Build history of the part. All positions in model axes, mm. Face numbers are marked on the shaded views. A direction names the side the tool comes from. Coordinates: 2 decimals unless noted, no trailing zeros. Order: outer loops, then holes, each group sorted by start corner. A loop starts at its lowest first (then second) coordinate and runs counter-clockwise, first axis right, second up. Notation, with made-up numbers: (-4, 36.5) - (38, 36.5) arc R17 ccw to (38, 41.5) - close; hole circle Ø4 at (17.5, 15.5). An arc over 180 degrees is marked (long way). Return JSON: item names as keys, results as strings.
from build123d import *

# Parameters (mm, degrees)
SKETCH1_W           = 457.2
SKETCH1_H           = 1244.6
BOSS_EXTRUDE1_DEPTH = 63.5
SKETCH4_W           = 457.2
SKETCH4_H           = 63.5
BOSS_EXTRUDE2_DEPTH = 266.7
CUT_EXTRUDE7_DEPTH  = 100.076
SKETCH12_W          = 63.5
SKETCH12_H          = 1244.6
CUT_EXTRUDE8_DEPTH  = 253.746


with BuildPart() as part:
    # Sketch1 → Boss-Extrude1 (new body)
    with BuildSketch(Plane(origin=(0, 0, 0), x_dir=(1, 0, 0), z_dir=(0, 1, 0))):
        with Locations((228.6, 622.3)):
            Rectangle(SKETCH1_W, SKETCH1_H)
    extrude(amount=BOSS_EXTRUDE1_DEPTH)

    # Sketch4 → Boss-Extrude2 (add)
    with BuildSketch(Plane(origin=(0, 63.5, 0), x_dir=(1, 0, 0), z_dir=(0, 1, 0))):
        with Locations((228.6, 1212.85)):
            Rectangle(SKETCH4_W, SKETCH4_H)
    boss_extrude2 = extrude(amount=BOSS_EXTRUDE2_DEPTH)

    # Mirror7: Boss-Extrude2 across plane
    add(boss_extrude2.mirror(Plane(origin=(0, 0, -622.3), x_dir=(1, 0, 0), z_dir=(0, 0, -1))))

    # Sketch11 → Cut-Extrude7 (cut)
    with BuildSketch(Plane.XY.offset(-1181.1)):
        Polygon((0, 63.5), (0, 330.2), (457.2, 330.2), (457.2, 229.907191107), align=None)
    cut_extrude7 = extrude(amount=-CUT_EXTRUDE7_DEPTH, mode=Mode.SUBTRACT)

    # Mirror8: Cut-Extrude7 across plane
    add(cut_extrude7.mirror(Plane(origin=(0, 0, -622.3), x_dir=(1, 0, 0), z_dir=(0, 0, -1))), mode=Mode.SUBTRACT)

    # Sketch12 → Cut-Extrude8 (cut)
    with BuildSketch(Plane.XZ):
        with Locations((31.75, -622.3)):
            Rectangle(SKETCH12_W, SKETCH12_H)
    extrude(amount=-CUT_EXTRUDE8_DEPTH, mode=Mode.SUBTRACT)


solid = part.part
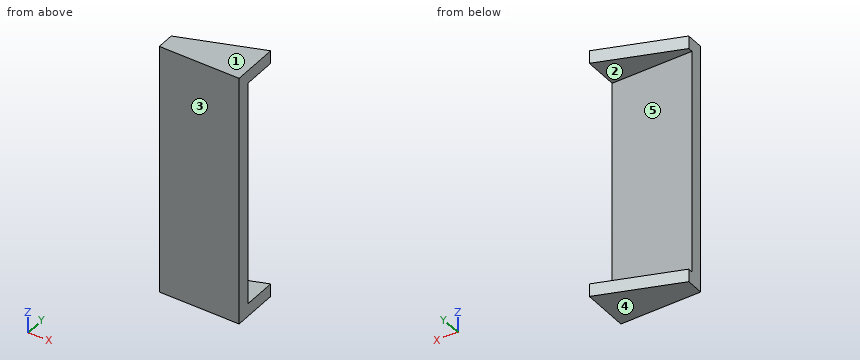
1. Cut at C-C on z = -311. Give the cut face in (x, y).
Check values:
{"outline": "(63.5, 0) - (457.2, 0) - (457.2, 63.5) - (63.5, 63.5) - close"}
2. Tool access for the marked faces 1 and 2: list every direction of +Z, -Z, +X, -X, +Y, -Y with a clear straight run to the whole face (end or side of a thin tool).
Check values:
{"face 1": "+Z, +X, -X, +Y, -Y", "face 2": "+X, -X, +Y"}
3. Cut at B-B on x = 370.5. Give the cut face in (y, z), plus the area to 3 significant figures.
Check values:
{"outline": "(0, -1244.6) - (198.35, -1244.6) - (198.35, -1181.1) - (63.5, -1181.1) - (63.5, -63.5) - (198.35, -63.5) - (198.35, 0) - (0, 0) - close", "area": "96,200 mm²"}
4. Cut at D-D on y = 108. Give the cut face in (x, z).
Check values:
{"outline": "(122.26, -1244.6) - (457.2, -1244.6) - (457.2, -1181.1) - (122.26, -1181.1) - close; (122.26, -63.5) - (457.2, -63.5) - (457.2, 0) - (122.26, 0) - close"}
5. Mould opens along Z. For the marked faces 3, 4 and 5 say: pulls with the +Z half, pulls with the -Z half, needs draft (parallel to the pull), parting line crosses it, or undercut.
Check values:
{"face 3": "needs draft", "face 4": "pulls with the -Z half", "face 5": "undercut"}
6. Cut at A-A on y = 173.5. Give the cut face in (x, z).
Check values:
{"outline": "(302.22, -1244.6) - (457.2, -1244.6) - (457.2, -1181.1) - (302.22, -1181.1) - close; (302.22, -63.5) - (457.2, -63.5) - (457.2, 0) - (302.22, 0) - close"}
7. Drop a flat-ended pin along its axis: pin 1 (2 mm diameter, centred on x = 150, z = -275, fed in from +Y). Give the stop position or say it passes through.
Check values:
{"pin 1": "y = 63.5"}
8. Probe L1, parallel to Z at x = 296.5, y = 90; L2, parallel to Y at x = 180, z = -468.5; L3, parallel to Y at x = 162, z = -1194.5. List the from-to ranges inside material, lowest first.
Check values:
{"L1": "-1244.6 to -1181.1, -63.5 to 0", "L2": "0 to 63.5", "L3": "0 to 122.46"}
